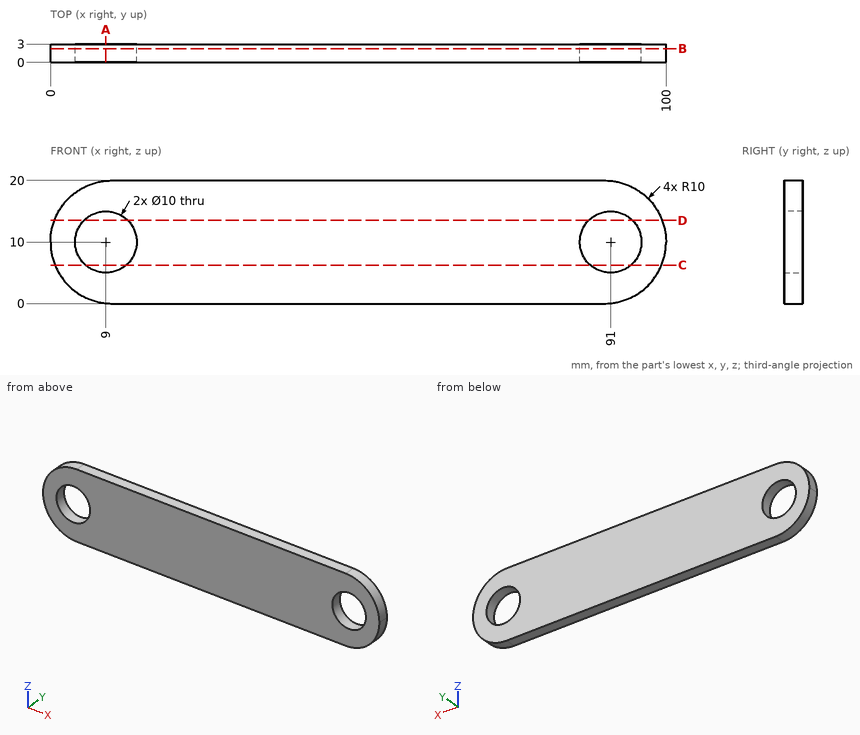
Geometry: see drawing. Coordinates: mm, zero at the bounding-box minimum. Coordinates: 2 decimals unless noted, no trailing zeros. Write each loop counter-clockwise with the first axis right and the second up, starting at its lowest first coordinate (ties: lowest second). Pieces come first, ordered by that corner, then holes. Notation, with made-up numbers: M 16,-5 L 52,-5 A22 ccw 52,8 Z; hole C 77.5,0.25 d3. An arc over 180 degrees is marked long. Answer as a JSON object with one key per item and string values.
1. Cut plane C-C on z = 6.25. Output: boundary loops of the cut face in (x, y), plus the area to 3 significant figures.
Evaluation:
{"outline": "M 0.73,0 L 5.69,0 L 5.69,3 L 0.73,3 Z; M 12.31,0 L 87.69,0 L 87.69,3 L 12.31,3 Z; M 94.31,0 L 99.27,0 L 99.27,3 L 94.31,3 Z", "area": "256 mm^2"}
2. Cut plane D-D on z = 13.5. Output: boundary loops of the cut face in (x, y), plus the area to 3 significant figures.
Evaluation:
{"outline": "M 0.63,0 L 5.43,0 L 5.43,3 L 0.63,3 Z; M 12.57,0 L 87.43,0 L 87.43,3 L 12.57,3 Z; M 94.57,0 L 99.37,0 L 99.37,3 L 94.57,3 Z", "area": "253 mm^2"}
3. Cut plane B-B on y = 2.25. State how many separate pieces and enclosed holes the cut face has, plus the area to 3 significant figures.
Evaluation:
{"separate pieces": "1", "enclosed holes": "2", "area": "1,760 mm^2"}
4. Cut plane A-A on x = 9. Output: boundary loops of the cut face in (y, z).
Evaluation:
{"outline": "M 0,0.05 L 3,0.05 L 3,5 L 0,5 Z; M 0,15 L 3,15 L 3,19.95 L 0,19.95 Z"}
5. Ray query, L1, parallel to X at y = 1.2, z = 10; L2, parallel to X at y = 2.6, z = 6.25; L3, parallel to Z at x = 8, y = 1.5. Return the intervals inside material, ascending.
Evaluation:
{"L1": "0 to 4, 14 to 86, 96 to 100", "L2": "0.73 to 5.69, 12.31 to 87.69, 94.31 to 99.27", "L3": "0.2 to 5.1, 14.9 to 19.8"}
